Design review of the part shown in the three views and the two pictorial views. Dimensions are in mm from the part's minimum x, y and z. Round coordinates to 2 decimals unless told otherwise and drop trailing zeros. Write each loop counter-clockwise with the first axis right and the second up, starting at its lowest first coordinate (ties: lowest second). Pieces come first, ordered by that corner, then holes. Notation, with made-up numbers: (57, 77.25) - (112, 77.25) arc R9 ccw to (112, 91.25) - close; hole circle Ø8 at (35, -32). An arc over 180 degrees is marked (long way). Use one line per item in the form item = value.
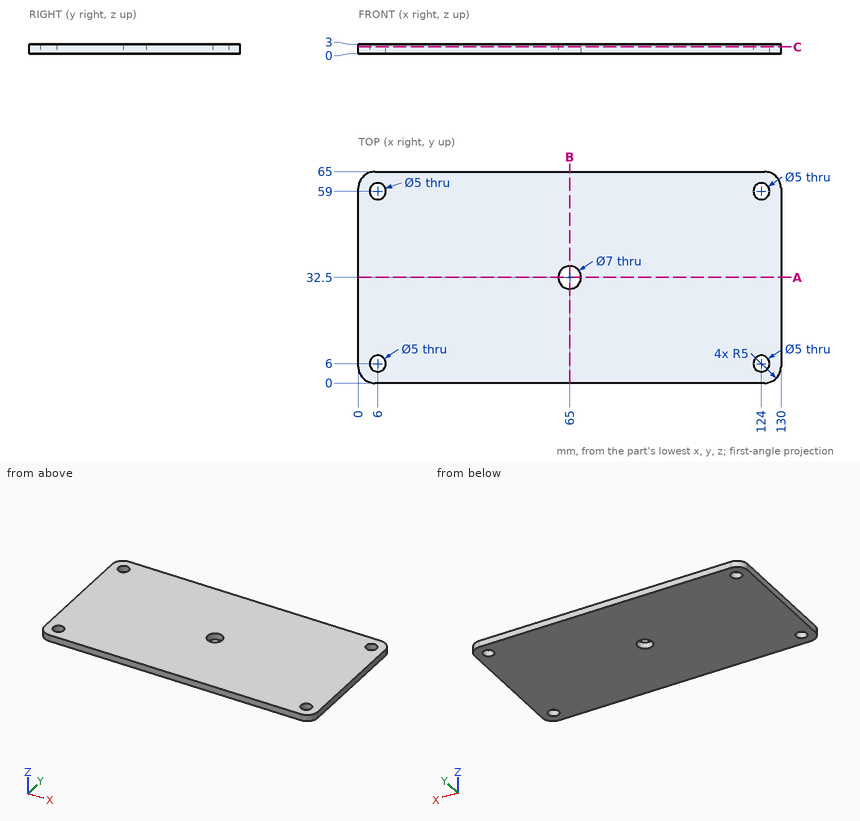
(1) Add section B-B on x = 65. Write out the cut boundary in (y, z), then the cut area to 3 significant figures.
Geometry results:
outline = (0, 0) - (29, 0) - (29, 3) - (0, 3) - close; (36, 0) - (65, 0) - (65, 3) - (36, 3) - close
area = 174 mm2
(2) Insertion check: P1, Ø8, axis at x = 124, y = 6, coming from the +Z side. The pin has a flat end and moves straight along its axis. Give the tip position at first contact, or say it passes through.
Geometry results:
P1 = 3
(3) Add section A-A on y = 32.5. Write out the cut boundary in (x, z), then the cut area to 3 significant figures.
Geometry results:
outline = (0, 0) - (61.5, 0) - (61.5, 3) - (0, 3) - close; (68.5, 0) - (130, 0) - (130, 3) - (68.5, 3) - close
area = 369 mm2
(4) Add section C-C on z = 2.15. Write out the cut boundary in (x, y), then the cut area to 3 significant figures.
Geometry results:
outline = (0, 5) arc R5 ccw to (5, 0) - (125, 0) arc R5 ccw to (130, 5) - (130, 60) arc R5 ccw to (125, 65) - (5, 65) arc R5 ccw to (0, 60) - close; hole circle Ø5 at (6, 6); hole circle Ø5 at (6, 59); hole circle Ø7 at (65, 32.5); hole circle Ø5 at (124, 6); hole circle Ø5 at (124, 59)
area = 8,310 mm2
(5) To check wall thickness, follow L1, parallel to Y at x = 6, z = 1.05; L2, parallel to Y at x = 63, z = 0.8; L3, parallel to X at y = 31, z = 0.75. State the ranges of each line that lie inside material, in increasing order.
Geometry results:
L1 = 0 to 3.5, 8.5 to 56.5, 61.5 to 65
L2 = 0 to 29.63, 35.37 to 65
L3 = 0 to 61.84, 68.16 to 130
